Can you work these out from the model? Positions are in its coordinate system, mm. A direction names the side the tool comes from. Coordinates: 2 decimals unless noted, no trailing zeros. Write each loop counter-clockwise with the first axis right and the second up, starting at its lowest first coordinate (ties: lowest second). Pieces come first, ordered by that corner, then holes. Notation, with made-up numbers: (75, -15.5) - (91, -15.5) arc R11 ccw to (91, -10.5) - close; hole circle Ø2 at (59.5, 34). An arc over 180 degrees is marked (long way). Use one line per item in the form item = value. Start each with the question number.
(1) On a 3-axis mill with a long thin cutter (end or side, diameter ignored), from which of +Z, -Z, +X, -X, +Y, -Y can I reach the whole of each face in a straight line? I mean faces 5 (the face through (-20, 0, 10)), 6 (the face through (-3, 28, 8)), 7 (the face through (-24, -3, 8)), 8 (the face through (-4.214, -13.378, 2.028)). Say none if no direction works.
(2) If we section it at C-C on z = 3: Please give me the cut outline in (x, y), then the cut area to 3 significant figures.
(3) If we section it at A-A on y = 0: Please give me the cut outline in (x, z), then the cut area to 3 significant figures.
(4) If we section it at D-D on x = -6.75: Please give me the cut outline in (y, z).
(5) For pin 1 Ø1 at (y, z) = (-13.5, 6) entering from -X; pin 2 Ø3 at (y, z) = (0, 13) entering from +X; pin 3 Ø8 at (y, z) = (0.5, 7) entering from -X; pin 4 Ø6 at (x, z) = (-15, 9.5) entering from -Y, each with a flat end and sliding along its axis, tell me the tip position at first contact or that it passes through.
(6) Thinking about a two-plate mould opening in Z: for faces 1 (the face through (-10, 0, 0)), 2 (the face through (-26, 1, 8)), 3 (the face through (-23.02, 0.05, 11.75)), 4 (the face through (-1.52, -26.82, 5.73)), which applies, pulls with the +Z half, pulls with the -Z half, needs draft (parallel to the pull), parting line crosses it, or undercut?
(7) If we section it at B-B on z = 7: Please give me the cut outline in (x, y).
(8) If I drill on probe 1 along Z at (x, y) = (-24.5, 0); probe 2 along Y at (x, z) = (-13, 1); probe 3 along Y at (x, z) = (-1.95, 7), over which ranges is the centre line in solid material (lowest first)? Write a range as from..to.
Autodesk Inventor part; units mm, degrees
ref_plane "YZ Plane" through (0, 0, 0) normal (1, 0, 0) x (0, 1, 0)
ref_plane "XZ Plane" through (0, 0, 0) normal (0, 1, 0) x (-1, 0, 0)
ref_plane "XY Plane" through (0, 0, 0) normal (0, 0, 1) x (1, 0, 0)
sketch "스케치1" plane through (0, 0, 0) normal (0, 0, 1) x (1, 0, 0)
  arc A0 (0, 5.2) -> (0, -5.2) centre (0, 0) ccw
  arc A1 (0, 23) -> (0, -23) centre (0, 0) ccw
  line L0 (0, 0) -> (0, 23)
  line L1 (0, 0) -> (0, -23)
  dimension "d0" = 10.4
  dimension "d1" = 46
extrude "돌출1" add sketch "스케치1" along normal blind 4 contours A0 L1 A1 L0
sketch "스케치2" plane through (0, 0, 4) normal (0, 0, 1) x (1, 0, 0)
  arc A0 (0, 20) -> (0, -20) centre (0, 0) ccw
  arc A1 (0, 23) -> (0, -23) centre (0, 0) ccw
  line L0 (0, 20) -> (0, 29)
  line L1 (0, 0) -> (0, -29)
  arc A2 (-3, -28.8444) -> (0, -29) centre (0, 0) ccw
  arc A3 (0, 29) -> (-3, 28.8444) centre (0, 0) ccw
  line L2 (-3, 28.8444) -> (-3, 19.7737)
  line L3 (-3, -19.7737) -> (-3, -22.8035)
  line L4 (-3, -28.8444) -> (-3, -19.7737)
  line L5 (-3, 19.7737) -> (-3, 28.8444)
  line L6 (-3, 22.8035) -> (-3, 19.7737)
  line L7 (-3, -19.7737) -> (-3, -28.8444)
  line L8 (0, -29) -> (0, -20)
  line L9 (0, 20) -> (0, 29)
  line L10 (0, 29) -> (0, 20)
  line L11 (0, -20) -> (0, -29)
  dimension "d4" = 40
  dimension "d5" = 46
  dimension "d6" = 29
  dimension "d7" = 29
extrude "돌출2" add sketch "스케치2" along normal blind 12
sketch "스케치3" plane through (-3, -28.8444, 4) normal (-1, 0, 0) x (0, 0, 1)
  line L0 (0, 51.6479) -> (12, 51.6479)
  line L1 (12, 57.6888) -> (12, 51.6479)
  line L2 (0, 57.6888) -> (12, 57.6888)
  line L3 (0, 57.6888) -> (0, 51.6479)
  line L4 (12, 6.0409) -> (0, 6.0409)
  line L5 (0, 6.0409) -> (0, 0)
  line L6 (0, 0) -> (12, 0)
  line L7 (12, 6.0409) -> (12, 0)
  circle A0 centre (9, 3) radius 1.6
  circle A1 centre (3, 3) radius 1.6
  circle A2 centre (9, 54.6888) radius 1.6
  circle A3 centre (3, 54.6888) radius 1.6
  point P0 (-4, 28.8444)
  dimension "d16" = 3.2
  dimension "d17" = 3.2
  dimension "d18" = 3.2
  dimension "d19" = 3.2
  dimension "d20" = 3
  dimension "d21" = 3
  dimension "d22" = 3
  dimension "d23" = 3
  dimension "d24" = 3
  dimension "d25" = 3
  dimension "d26" = 3
  dimension "d27" = 3
extrude "돌출3" cut sketch "스케치3" against normal up to surface (3 mm away) contours A0 | A1 | A2 | A3
sketch "스케치4" plane through (0, 0, 4) normal (0, 0, 1) x (1, 0, 0)
  circle A0 centre (-5.7403, 13.8582) radius 1.25
  circle A1 centre (-5.7403, -13.8582) radius 1.25
  circle A2 centre (-13.8582, -5.7403) radius 1.25
  circle A3 centre (-13.8582, 5.7403) radius 1.25
  line L0 (-0.7301, 13.7687) -> (-0.7301, 13.7687)
  circle A4 centre (-5.7403, 13.8582) radius 1.6
  circle A5 centre (-13.8582, 5.7403) radius 1.6
  circle A6 centre (-13.8582, -5.7403) radius 1.6
  circle A7 centre (-5.7403, -13.8582) radius 1.6
  arc A8 (0, 20) -> (0, -20) centre (0, 0) ccw
  line L1 (0, -20) -> (0, -5.2)
  arc A9 (0, 5.2) -> (0, -5.2) centre (0, 0) ccw
  line L2 (0, 5.2) -> (0, 20)
  line L3 (0, 0) -> (-5.7403, 13.8582)
  line L4 (0, 0) -> (15, 0) construction
  line L5 (0, 0) -> (-13.8582, 5.7403)
  line L6 (0, 0) -> (15, 0) construction
  line L7 (0, 0) -> (-13.8582, 5.7403)
  line L8 (0, 0) -> (15, 0) construction
  line L9 (0, 0) -> (-13.8582, -5.7403)
  line L10 (0, 0) -> (15, 0) construction
  line L11 (0, 0) -> (-5.7403, -13.8582)
  line L12 (0, 0) -> (15, 0) construction
  dimension "d30" = 3.2
  dimension "d31" = 3.2
  dimension "d32" = 3.2
  dimension "d33" = 3.2
  dimension "d56" = 15
  dimension "d57" = 112.5
  dimension "d58" = 15
  dimension "d59" = 157.5
  dimension "d61" = 15
  dimension "d62" = 202.5
  dimension "d63" = 15
  dimension "d64" = 157.5
  dimension "d65" = 15
  dimension "d66" = 112.5
extrude "돌출4" cut sketch "스케치4" against normal up to surface (4 mm away) contours A0 | A4 | A1 | A7 | A2 | A6 | A3 | A5
sketch "스케치5" plane through (0, 0, 16) normal (0, 0, 1) x (1, 0, 0)
  circle A0 centre (0, 0) radius 23
  arc A1 (-3, 22.8035) -> (-3, -22.8035) centre (0, 0) ccw
  line L0 (-23, 0) -> (-26, 0)
  line L1 (-23, 0) -> (-20, 0) construction
  line L2 (-26, 0) -> (-26, -3)
  line L3 (-26, -3) -> (-22.8035, -3)
  line L4 (-26, 0) -> (-26, 3)
  line L5 (-26, 0) -> (-23, 0) construction
  line L6 (-26, 3) -> (-22.8035, 3)
  dimension "d36" = 46
  dimension "d37" = 3
  dimension "d38" = 180
  dimension "d39" = 3
  dimension "d40" = 90
  dimension "d41" = 90
  dimension "d42" = 3
  dimension "d43" = 90
extrude "돌출5" add sketch "스케치5" against normal blind 16 contours A0 L0 L4 L6 | L3 L2 L0 A0
sketch "스케치6" plane through (-26, -3, 16) normal (-1, 0, 0) x (0, 0, 1)
  line L0 (0, 6) -> (0, 0)
  line L1 (0, 6) -> (-16, 6)
  line L2 (-16, 0) -> (-16, 6)
  line L3 (0, 0) -> (-16, 0)
  circle A0 centre (-3, 3) radius 1.25
  circle A1 centre (-9, 3) radius 1.25
  point P0 (-16, 3)
  dimension "d46" = 2.5
  dimension "d47" = 2.5
  dimension "d48" = 3
  dimension "d49" = 7
  dimension "d50" = 3
  dimension "d51" = 3
extrude "돌출6" cut sketch "스케치6" against normal blind 8 contours A0 | A1
sketch "스케치7" plane through (0, 0, 0) normal (0, 0, -1) x (-1, 0, 0)
  arc A0 (0, -23) -> (3, -22.8035) centre (0, 0) ccw
  line L0 (0, -29) -> (0, -23)
  arc A1 (0, -29) -> (3, -28.8444) centre (0, 0) ccw
  line L1 (3, -22.8035) -> (3, -28.8444)
  arc A2 (3, 22.8035) -> (0, 23) centre (0, 0) ccw
  line L2 (3, 28.8444) -> (3, 22.8035)
  arc A3 (3, 28.8444) -> (0, 29) centre (0, 0) ccw
  line L3 (0, 23) -> (0, 29)
extrude "돌출7" add sketch "스케치7" against normal blind 4
properties part number "조인트3링크2고정부" material "알루미늄 6061"
Reported:
q1.face_5 = +Z, +X
q1.face_6 = +Z, -Z, -X, +Y
q1.face_7 = +Z, -Z, -X, -Y
q1.face_8 = +Z, -Z
q2.outline = (-26, -3) - (-22.8, -3) arc R23 ccw to (-3, -22.8) - (-3, -28.84) arc R29 ccw to (0, -29) - (0, -5.2) arc R5.2 cw to (0, 5.2) - (0, 29) arc R29 ccw to (-3, 28.84) - (-3, 22.8) arc R23 ccw to (-22.8, 3) - (-26, 3) - close; hole circle Ø3.2 at (-13.86, -5.74); hole circle Ø3.2 at (-13.86, 5.74); hole circle Ø3.2 at (-5.74, -13.86); hole circle Ø3.2 at (-5.74, 13.86)
q2.area = 811 mm2
q3.outline = (-26, 0) - (-5.2, 0) - (-5.2, 4) - (-20, 4) - (-20, 5.75) - (-26, 5.75) - close; (-26, 8.25) - (-20, 8.25) - (-20, 11.75) - (-26, 11.75) - close; (-26, 14.25) - (-20, 14.25) - (-20, 16) - (-26, 16) - close
q3.area = 125 mm2
q4.outline = (-21.99, 0) - (-15.1, 0) - (-15.1, 4) - (-18.83, 4) - (-18.83, 16) - (-21.99, 16) - close; (-12.62, 0) - (12.62, 0) - (12.62, 4) - (-12.62, 4) - close; (15.1, 0) - (21.99, 0) - (21.99, 16) - (18.83, 16) - (18.83, 4) - (15.1, 4) - close
q5.pin_1 = -18.97
q5.pin_2 = -19.94
q5.pin_3 = -26
q5.pin_4 = -19.62
q6.face_1 = pulls with the -Z half
q6.face_2 = needs draft
q6.face_3 = undercut
q6.face_4 = undercut
q7.outline = (-26, -3) - (-22.8, -3) arc R23 ccw to (-3, -22.8) - (-3, -24.24) - (0, -24.24) - (0, -20) arc R20 cw to (-19.96, -1.25) - (-26, -1.25) - close; (-26, 1.25) - (-19.96, 1.25) arc R20 cw to (0, 20) - (0, 24.24) - (-3, 24.24) - (-3, 22.8) arc R23 ccw to (-22.8, 3) - (-26, 3) - close; (-3, -28.84) arc R29 ccw to (0, -29) - (0, -27.44) - (-3, -27.44) - close; (-3, 27.44) - (0, 27.44) - (0, 29) arc R29 ccw to (-3, 28.84) - close
q8.probe_1 = 0..5.75, 8.25..11.75, 14.25..16
q8.probe_2 = -18.97..-7.09, -4.39..4.39, 7.09..18.97
q8.probe_3 = -28.93..-27.44, -24.24..-19.9, 19.9..24.24, 27.44..28.93
